Read the model definition and answer for the solid it produces. Units are mm, in the model's axes. Give positions to 0.01 mm unless a question says otherwise; leave off trailing zeros. Write each loop counter-clockwise with the first axis right and the second up, starting at its lowest first coordinate (ties: lowest second). Pieces come first, ordered by that corner, then holes. Notation, with made-up numbers: (87, -32) -> (100, -32) arc R19 ccw to (100, -14) -> close; hole circle Ø2 at (78.5, 86). An arc over 180 degrees is marked (long way). Use a Markdown table: item, result.
from build123d import *

# Parameters (mm, degrees)
F1_DEPTH = 18
F3_D     = 8
F3_DEPTH = 16
F3_TIP   = 2.4034424761


with BuildPart() as f1:
    # F0 (on Front) → F1 (new body)
    with BuildSketch(Plane.XZ):
        with BuildLine():
            Line((400, 0), (0, 0))
            Line((0, 0), (0, -100))
            Line((0, -100), (37, -100))
            Line((37, -100), (45.1614643503, -53.7140356084))
            ThreePointArc((45.1614643503, -53.7140356084), (43.9616795743, -48.3021562165), (48.6368321424, -51.2805568824))
            Line((48.6368321424, -51.2805568824), (60.4545251785, -53.3643350144))
            Line((60.4545251785, -53.3643350144), (61.0056646383, -50.2386678164))
            ThreePointArc((61.0056646383, -50.2386678164), (64.4810324303, -47.8051890904), (66.9145111563, -51.2805568824))
            Line((66.9145111563, -51.2805568824), (78.7322041925, -53.3643350144))
            ThreePointArc((78.7322041925, -53.3643350144), (84.1440835844, -52.1645502383), (81.1656829185, -56.8397028064))
            Line((81.1656829185, -56.8397028064), (73.5553580279, -100))
            Line((73.5553580279, -100), (326.4446419721, -100))
            Line((326.4446419721, -100), (318.8343170815, -56.8397028064))
            ThreePointArc((318.8343170815, -56.8397028064), (315.8559164156, -52.1645502383), (321.2677958075, -53.3643350144))
            Line((321.2677958075, -53.3643350144), (333.0854888437, -51.2805568824))
            ThreePointArc((333.0854888437, -51.2805568824), (335.5189675697, -47.8051890904), (338.9943353617, -50.2386678164))
            Line((338.9943353617, -50.2386678164), (339.5454748215, -53.3643350144))
            Line((339.5454748215, -53.3643350144), (351.3631678576, -51.2805568824))
            ThreePointArc((351.3631678576, -51.2805568824), (356.0383204257, -48.3021562165), (354.8385356497, -53.7140356084))
            Line((354.8385356497, -53.7140356084), (363, -100))
            Line((363, -100), (400, -100))
            Line((400, -100), (400, 0))
        make_face()
    extrude(amount=F1_DEPTH)

    # F3
    with Locations(Plane.XY):
        with Locations((75, -9), (325, -9)):
            Hole(F3_D / 2, depth=F3_DEPTH)
            with Locations((0, 0, -(F3_DEPTH + F3_TIP / 2))):  # 118° drill point
                Cone(0, F3_D / 2, F3_TIP, mode=Mode.SUBTRACT)


solid = f1.part
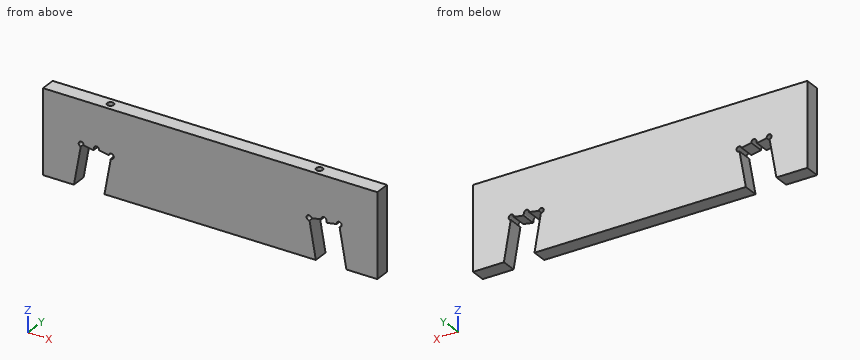
Item 1: A cutting plane is placed at A-A (z = -72). Give the vertices of the cut face in (x, y).
Return value:
| item | result |
|---|---|
| outline | (0, -18) -> (41.94, -18) -> (41.94, 0) -> (0, 0) -> close; (78.49, -18) -> (321.51, -18) -> (321.51, 0) -> (78.49, 0) -> close; (358.06, -18) -> (400, -18) -> (400, 0) -> (358.06, 0) -> close |
Item 2: This flat-tipped pin is pushed along its axis until it touches: P1, Ø6, axis at x = 53, z = -25, coming from the +Y side. Where does it stop, or does it pass through?
Return value:
| item | result |
|---|---|
| P1 | y = 0 |
Item 3: A cutting plane is placed at B-B (x = 56). Give the vertices of the cut face in (y, z), then the cut area to 3 significant figures.
Return value:
| item | result |
|---|---|
| outline | (-18, -52.58) -> (0, -52.58) -> (0, 0) -> (-18, 0) -> close |
| area | 946 mm^2 |
Item 4: Straight lines are drawn through the part: line 1 along X through (y, z) = (-9, -12.25); line 2 along Y through (x, z) = (325, -6); line 3 along X through (y, z) = (-16.5, -66). For each, find the intervals that lie inside material, in ascending order. Write a range as [from, to].
Return value:
| item | result |
|---|---|
| line 1 | [0, 71], [79, 321], [329, 400] |
| line 2 | [-18, -13], [-5, 0] |
| line 3 | [0, 43], [79.55, 320.45], [357, 400] |
